Check sheet for the drawn part. Datum: minimum x, y, z corner. Units: mm. Give positions to 0.01 mm unless a question says otherwise; leave off trailing zeros. Loops run counter-clockwise (first coordinate to the right, second up) from the corner with the lowest first, then second, coordinate; pieces in that order, holes last. Notation, with made-up numbers: (-12.5, 6) -> (16.5, 6) arc R19 ccw to (16.5, 42) -> close; hole circle Ø6 at (55, 12). An arc over 180 degrees is marked (long way). One line per question, with ' | ' between items.
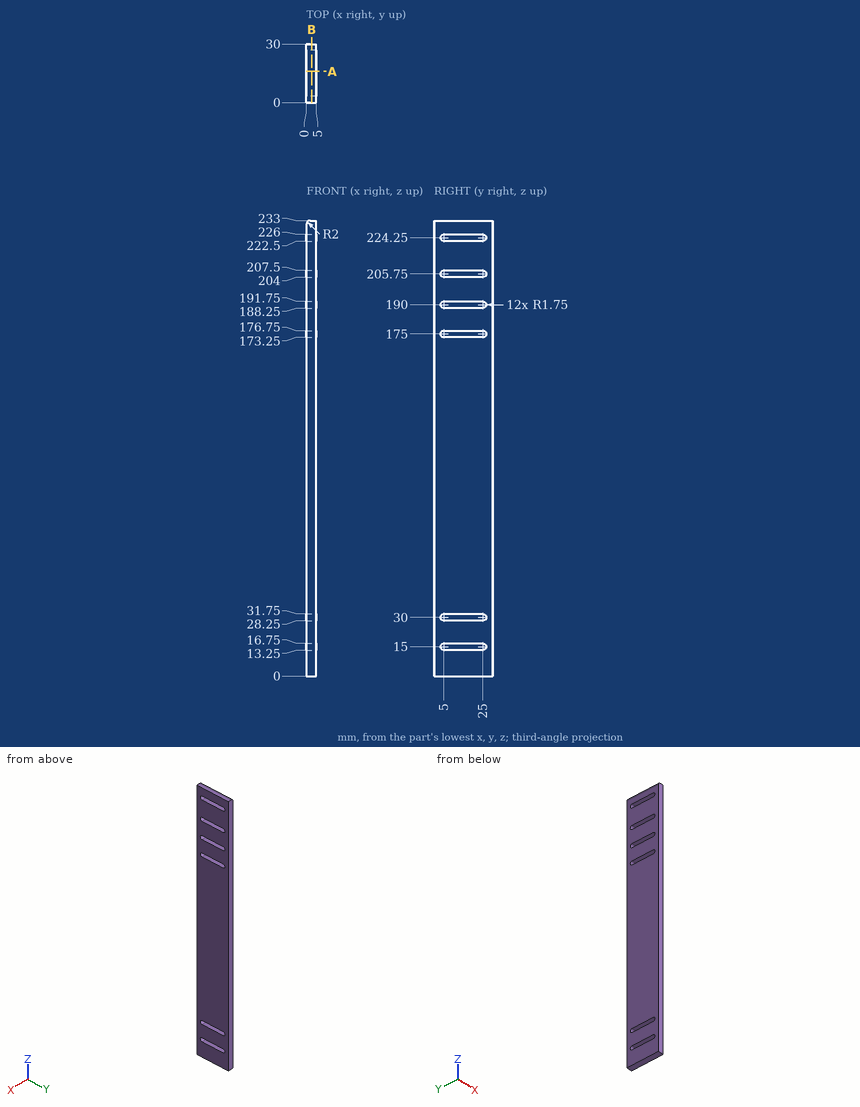
Item 1: Scan line: probe 1 along Y at (x, z) = (3.5, 30). Record every from-to range of solid material in increasing order.
Result:
probe 1: 0 to 3.25, 26.75 to 30
Item 2: Sectioned sample at A-A (y = 16). Give the number of separate pieces and of enclosed holes in the cut face, plus the area to 3 significant figures.
Result:
separate pieces: 7 | enclosed holes: 0 | area: 1,060 mm2
Item 3: Sectioned sample at B-B (x = 2.75). Record the cut outline in (y, z).
Result:
outline: (0, 0) -> (30, 0) -> (30, 233) -> (0, 233) -> close; hole (5, 13.25) -> (25, 13.25) arc R1.75 ccw to (25, 16.75) -> (5, 16.75) arc R1.75 ccw to start; hole (5, 28.25) -> (25, 28.25) arc R1.75 ccw to (25, 31.75) -> (5, 31.75) arc R1.75 ccw to start; hole (5, 173.25) -> (25, 173.25) arc R1.75 ccw to (25, 176.75) -> (5, 176.75) arc R1.75 ccw to start; hole (5, 188.25) -> (25, 188.25) arc R1.75 ccw to (25, 191.75) -> (5, 191.75) arc R1.75 ccw to start; hole (5, 204) -> (25, 204) arc R1.75 ccw to (25, 207.5) -> (5, 207.5) arc R1.75 ccw to start; hole (5, 222.5) -> (25, 222.5) arc R1.75 ccw to (25, 226) -> (5, 226) arc R1.75 ccw to start
